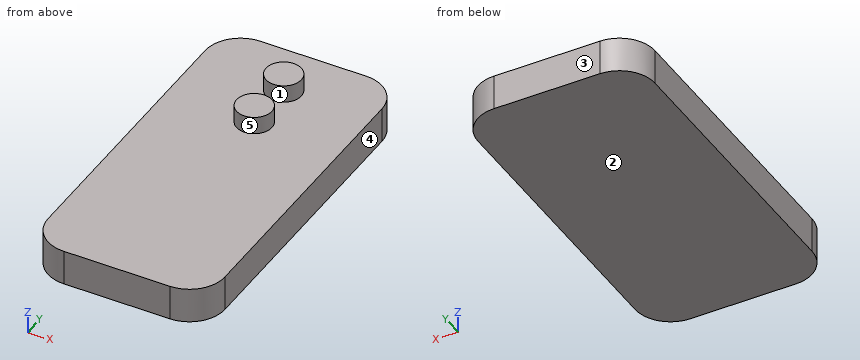
from build123d import *

# Parameters (mm, degrees)
BOSS_EXTRU_1_DEPTH = 10
ESQUISSE2_R        = 5
BOSS_EXTRU_2_DEPTH = 5


with BuildPart() as part:
    # Esquisse1 → Boss.-Extru.1 (new body)
    with BuildSketch(Plane.XY):
        with BuildLine():
            Line((-15, 0), (15, 0))
            ThreePointArc((15, 0), (22.071067812, 2.928932188), (25, 10))
            Line((25, 10), (25, 90))
            ThreePointArc((25, 90), (22.071067812, 97.071067812), (15, 100))
            Line((15, 100), (-15, 100))
            ThreePointArc((-15, 100), (-22.071067812, 97.071067812), (-25, 90))
            Line((-25, 90), (-25, 10))
            ThreePointArc((-25, 10), (-22.071067812, 2.928932188), (-15, 0))
        make_face()
    extrude(amount=BOSS_EXTRU_1_DEPTH)

    # Esquisse2 → Boss.-Extru.2 (add)
    with BuildSketch(Plane.XY.offset(10)):
        with Locations(Location((0, 85, 0), (0, 0, 180))):
            Circle(ESQUISSE2_R)
        with Locations(Location((0, 70, 0), (0, 0, 180))):
            Circle(ESQUISSE2_R)
    extrude(amount=BOSS_EXTRU_2_DEPTH)


solid = part.part
Source: CAD feature listing. Evaluate the final solid. Frame: model axes, mm. Face numbers are marked on the shaded views. A direction names the side the tool comes from. Give positions to 0.01 mm unless a question says otherwise; leave off trailing zeros. Loops run counter-clockwise (first coordinate to the right, second up) from the corner with the lowest first, then second, coordinate; pieces in that order, holes last. Notation, with made-up numbers: (88.5, 67) -> (144.5, 67) arc R24 ccw to (144.5, 86) -> close; hole circle Ø11 at (15, -1.5). An arc over 180 degrees is marked (long way). Use a Markdown table: item, result. Add a question column.
1) First-contact query: pin 1 (10 mm diameter, centred on x = -4, y = 15.5, fed in from -Z); pin 2 (12 mm diameter, centred on x = 6, y = 53, fed in from +Z). Flat tips, straight axial feed; report the tip coordinate or a pass-through.
2) Section query A-A, the plane y = 85. Return the cut outline in (x, z).
3) Pull-direction query (Y, two-part tool) for the marked faces 3, 4 and 5; classes: +Y half, -Y half, draft (parallel to the pull), parting line (faces both ways), or undercut.
4) Section query C-C, the plane x = -4. Return the cut outline in (y, z).
5) Reachability of the marked faces 1 and 2 from +Z, -Z, +X, -X, +Y, -Y: full face, straight path, thin tool, end or side. Return the list, or none.
6) Section query B-B, the plane z = 7. Return the cut outline in (x, y), then the cut area to 3 significant figures.
7) Line query: line 1 along Z through (x, y) = (19, 87); line 2 along Y through (x, z) = (15.5, 5); line 3 along Y through (x, z) = (4.5, 10.25). Output: solid intervals per line, ascending. Write a range as [from, to].
8) Section query D-D, the plane y = 38.5. Return the cut outline in (x, z).
Numbers:
| question | item | result |
|---|---|---|
| 1 | pin 1 | stops at z = 0 |
| 1 | pin 2 | stops at z = 10 |
| 2 | outline | (-25, 0) -> (25, 0) -> (25, 10) -> (5, 10) -> (5, 15) -> (-5, 15) -> (-5, 10) -> (-25, 10) -> close |
| 3 | face 3 | +Y half |
| 3 | face 4 | draft |
| 3 | face 5 | undercut |
| 4 | outline | (0, 0) -> (100, 0) -> (100, 10) -> (88, 10) -> (88, 15) -> (82, 15) -> (82, 10) -> (73, 10) -> (73, 15) -> (67, 15) -> (67, 10) -> (0, 10) -> close |
| 5 | face 1 | +Z |
| 5 | face 2 | -Z, +X, -X, +Y, -Y |
| 6 | outline | (-25, 10) arc R10 ccw to (-15, 0) -> (15, 0) arc R10 ccw to (25, 10) -> (25, 90) arc R10 ccw to (15, 100) -> (-15, 100) arc R10 ccw to (-25, 90) -> close |
| 6 | area | 4,910 mm2 |
| 7 | line 1 | z = [0, 10] |
| 7 | line 2 | y = [0.01, 99.99] |
| 7 | line 3 | y = [67.82, 72.18], [82.82, 87.18] |
| 8 | outline | (-25, 0) -> (25, 0) -> (25, 10) -> (-25, 10) -> close |
